from build123d import *

# Parameters (mm, degrees)
F1_DEPTH = 5


with BuildPart() as f1:
    # F0 (on Front) → F1 (new body, symmetric)
    with BuildSketch(Plane.XZ):
        with BuildLine():
            ThreePointArc((-0.625, 0), (-1.06434, 1.06066), (-2.125, 1.5))
            Line((-2.125, 1.5), (-2.125, 0.25))
            ThreePointArc((-2.125, 0.25), (-1.948223, 0.176777), (-1.875, 0))
            ThreePointArc((-1.875, 0), (-1.948223, -0.176777), (-2.125, -0.25))
            Line((-2.125, -0.25), (-2.125, -1.5))
            ThreePointArc((-2.125, -1.5), (-1.06434, -1.06066), (-0.625, 0))
        make_face()
        with BuildLine():
            Line((-2.125, 0.25), (-2.125, 1.5))
            ThreePointArc((-2.125, 1.5), (-3.625, 0), (-2.125, -1.5))
            Line((-2.125, -1.5), (-2.125, -0.25))
            ThreePointArc((-2.125, -0.25), (-2.375, 0), (-2.125, 0.25))
        make_face()
        with BuildLine():
            Line((2.125, 1.5), (-2.125, 1.5))
            ThreePointArc((-2.125, 1.5), (-1.06434, 1.06066), (-0.625, 0))
            ThreePointArc((-0.625, 0), (-1.06434, -1.06066), (-2.125, -1.5))
            Line((-2.125, -1.5), (2.125, -1.5))
            ThreePointArc((2.125, -1.5), (0.625, 0), (2.125, 1.5))
        make_face()
        with BuildLine():
            ThreePointArc((3.625, 0), (3.18566, 1.06066), (2.125, 1.5))
            Line((2.125, 1.5), (2.125, 0.25))
            ThreePointArc((2.125, 0.25), (2.301777, 0.176777), (2.375, 0))
            ThreePointArc((2.375, 0), (2.301777, -0.176777), (2.125, -0.25))
            Line((2.125, -0.25), (2.125, -1.5))
            ThreePointArc((2.125, -1.5), (3.18566, -1.06066), (3.625, 0))
        make_face()
        with BuildLine():
            Line((2.125, 0.25), (2.125, 1.5))
            ThreePointArc((2.125, 1.5), (0.625, 0), (2.125, -1.5))
            Line((2.125, -1.5), (2.125, -0.25))
            ThreePointArc((2.125, -0.25), (1.875, 0), (2.125, 0.25))
        make_face()
    extrude(amount=F1_DEPTH, both=True)


solid = f1.part
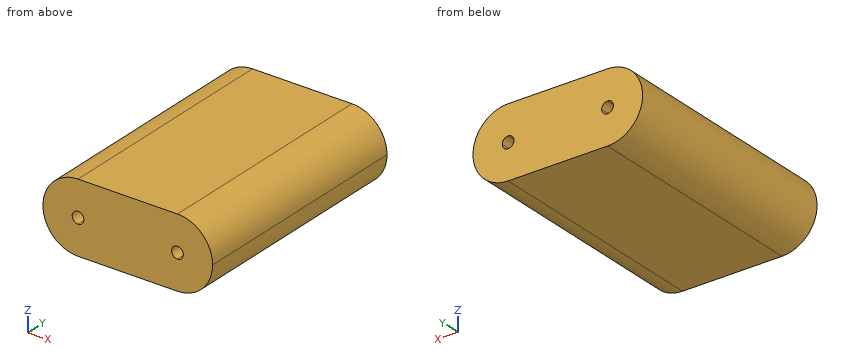
Source: CAD feature listing. Evaluate the final solid. Frame: model axes, mm. Coordinates: 2 decimals unless noted, no trailing zeros. Loops run counter-clockwise (first coordinate to the right, second up) from the corner with the lowest first, then second, coordinate; pieces in that order, holes last. Notation, with made-up numbers: (-1, -11) - (21, -11) arc R20 cw to (21, -5) - close; hole circle Ø6 at (-23, 88.25). An arc over 180 degrees is marked (long way). One line per question, with ' | ' between items.
1) Section A-A, the plane y = -1. Return loops of the section in (x, z) (3 decimals).
Report:
outline: (-2.125, -1.5) - (2.125, -1.5) arc R1.5 ccw to (3.625, 0) arc R1.5 ccw to (2.125, 1.5) - (-2.125, 1.5) arc R1.5 ccw to start; hole (-2.125, -0.25) arc R0.25 ccw to (-1.875, 0) arc R0.25 ccw to (-2.125, 0.25) arc R0.25 ccw to start; hole (2.125, -0.25) arc R0.25 ccw to (2.375, 0) arc R0.25 ccw to (2.125, 0.25) arc R0.25 ccw to start
2) Section C-C, the plane z = 0.9. Return loops of the section in (x, y) (3 decimals), then the cut area to 3 significant figures.
Report:
outline: (-3.325, -5) - (3.325, -5) - (3.325, 5) - (-3.325, 5) - close | area: 66.5 mm²
3) Line query: line 1 along X through (y, z) = (-3.5, -0.05); line 2 along Z through (x, y) = (2.5, 0.5); line 3 along Z through (x, y) = (-2.25, 4.75). Output: solid intervals per line, ascending.
Report:
line 1: x = -3.62 to -2.37, -1.88 to 1.88, 2.37 to 3.62 | line 2: z = -1.45 to 1.45 | line 3: z = -1.49 to -0.22, 0.22 to 1.49
4) First-contact query: P1, Ø1, axis at y = 0, z = 1, coming from the +X side. Flat tip, straight axial feed; report the tip coordinate or a pass-through.
Report:
P1: stops at x = 3.54
5) Section B-B, the plane x = -2.5. Return loops of the section in (y, z), then the cut area to 3 significant figures.
Report:
outline: (-5, -1.45) - (5, -1.45) - (5, 1.45) - (-5, 1.45) - close | area: 29.0 mm²
